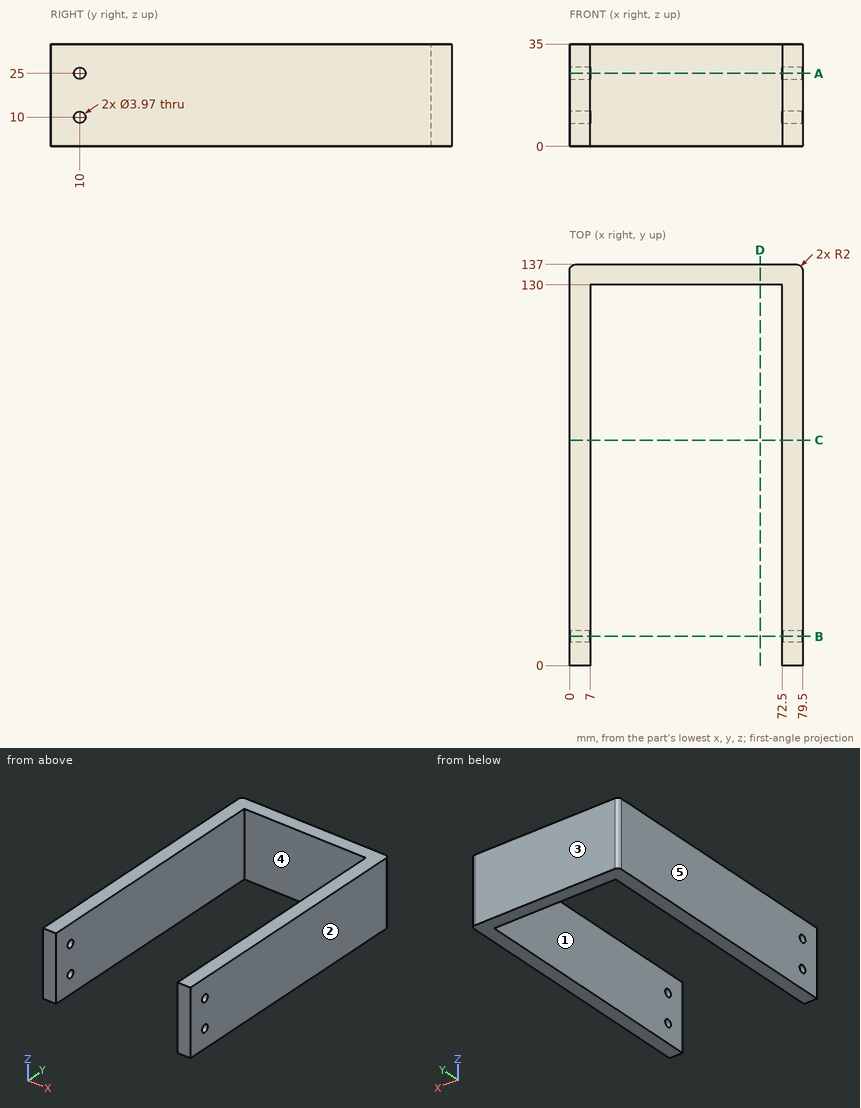
Verification items for this drawing (mm, ordinates from the low corner). A direction names the side the tool comes from. Give positions to 0.01 mm unless a question says otherwise; leave off trailing zeros. Loops run counter-clockwise (first coordinate to the right, second up) from the corner with the lowest first, then second, coordinate; pieces in that order, holes last. Notation, with made-up numbers: M 5,1 L 19,1 A35 cw 19,33 Z; hole C -28.5,33.25 d1. An arc over 180 degrees is marked long. Answer as a JSON object with one key per item and string values. Group by question number.
Q1. Release check for a two-part mould opening along X. For the marked faces 1, 2 and 3 record: released by +X, released by -X, zero draft, split by the parting line, or undercut.
Q2. Go/stop test with flat-tipped pins: P1, Ø2.5, axis at y = 10, z = 25, coming from the -X side; P2, Ø17.5, axis at x = 34, z = 24.5, coming from the -Y side. Record where each tip stops, or that it passes through.
Q3. Cross-section at D-D on x = 65. Record the cut outline in (y, z).
Q4. Cross-section at A-A on z = 25. Record the cut outline in (x, y) (3 decimals), then the cut area to 3 significant figures.
Q5. Cross-section at C-C on y = 77. Record the cut outline in (x, z), then the cut area to 3 significant figures.
Q6. Material ranges on line 1 along Z through (x, y) = (3.5, 10) (3 decimals); line 2 along X through (y, z) = (53.5, 4.5); line 3 along Y through (x, z) = (74.5, 25) (3 decimals), recorded low to high. Write a range as [from, to].
Q7. Cross-section at B-B on y = 10. Record the cut outline in (x, z) (3 decimals).
Q8. Access from +Z, -Z, +X, -X, +Y, -Y to the whole of each face (thin tool, end or side, straight path). Record for the marked faces 4 and 5.
Evaluation:
{
 "1": {"face 1": "undercut", "face 2": "released by +X", "face 3": "zero draft"},
 "2": {"P1": "passes through", "P2": "stops at y = 130"},
 "3": {"outline": "M 130,0 L 137,0 L 137,35 L 130,35 Z"},
 "4": {"outline": "M 0,0 L 7,0 L 7,8.015 L 0,8.015 Z; M 0,11.985 L 7,11.985 L 7,130 L 72.5,130 L 72.5,11.985 L 79.5,11.985 L 79.5,135 A2 ccw 77.5,137 L 2,137 A2 ccw 0,135 Z; M 72.5,0 L 79.5,0 L 79.5,8.015 L 72.5,8.015 Z", "area": "2,320 mm2"},
 "5": {"outline": "M 0,0 L 7,0 L 7,35 L 0,35 Z; M 72.5,0 L 79.5,0 L 79.5,35 L 72.5,35 Z", "area": "490 mm2"},
 "6": {"line 1": "z = [0, 8.015], [11.985, 23.015], [26.985, 35]", "line 2": "x = [0, 7], [72.5, 79.5]", "line 3": "y = [0, 8.015], [11.985, 137]"},
 "7": {"outline": "M 0,0 L 7,0 L 7,8.015 L 0,8.015 Z; M 0,11.985 L 7,11.985 L 7,23.015 L 0,23.015 Z; M 0,26.985 L 7,26.985 L 7,35 L 0,35 Z; M 72.5,0 L 79.5,0 L 79.5,8.015 L 72.5,8.015 Z; M 72.5,11.985 L 79.5,11.985 L 79.5,23.015 L 72.5,23.015 Z; M 72.5,26.985 L 79.5,26.985 L 79.5,35 L 72.5,35 Z"},
 "8": {"face 4": "+Z, -Z, -Y", "face 5": "+Z, -Z, -X, +Y, -Y"}
}
